Design review of the part built by this model. Coordinates are the model's own, in mm. Face numbers are marked on the shaded views. A direction names the side the tool comes from. Give positions to 0.01 mm unless a question says otherwise; leave off trailing zeros. Loops run counter-clockwise (first coordinate to the right, second up) from the corner with the lowest first, then second, coordinate; pieces in that order, holes last.
Autodesk Inventor part; units mm, degrees
ref_plane "YZ Plane" through (0, 0, 0) normal (1, 0, 0) x (0, 1, 0)
ref_plane "XZ Plane" through (0, 0, 0) normal (0, 1, 0) x (-1, 0, 0)
ref_plane "XY Plane" through (0, 0, 0) normal (0, 0, 1) x (1, 0, 0)
sketch "Sketch1" plane through (0, 0, 0) normal (0, 0, 1) x (1, 0, 0)
  arc A0 (1.7145, 0) -> (-1.7145, 0) centre (0, 0) ccw
  arc A1 (38.0096, -20.955) -> (34.5806, -20.955) centre (36.2951, -20.955) ccw
  line L0 (0, 0) -> (36.5724, 0) construction
  line L1 (-1.7145, 0) -> (-1.7145, -3.0427)
  line L2 (1.7145, 0) -> (1.7145, -3.0427)
  line L3 (34.5806, -20.955) -> (34.5806, -23.9977)
  line L4 (38.0096, -20.955) -> (38.0096, -23.9977)
  line L5 (0, 0) -> (0, -41.91) construction
  arc A2 (29.1702, -5.2325) -> (5.0807, 4.6768) centre (0, -41.91) ccw
  arc A3 (5.0807, 4.6768) -> (-2.0016, 2.862) centre (3.9541, -5.6536) ccw
  arc A4 (39.5833, -19.7781) -> (29.1702, -5.2325) centre (8.8547, -30.7765) ccw
  arc A5 (4.8053, 2.1517) -> (2.7829, 2.1102) centre (3.9541, -5.6536) ccw
  arc A6 (27.5892, -7.2205) -> (4.8053, 2.1517) centre (0, -41.91) ccw
  arc A7 (35.8607, -17.4896) -> (27.5892, -7.2205) centre (8.8547, -30.7765) ccw
  arc A8 (35.8607, -17.4896) -> (34.5806, -23.9977) centre (36.2951, -20.955) ccw
  arc A9 (38.0096, -23.9977) -> (39.5833, -19.7781) centre (36.2951, -20.955) ccw
  arc A10 (-2.0016, 2.862) -> (-1.7145, -3.0427) centre (0, 0) ccw
  arc A11 (1.7145, -3.0427) -> (2.7829, 2.1102) centre (0, 0) ccw
  line L6 (0, 0) -> (36.2951, -20.955) construction
  line L7 (12.8786, -1.5696) -> (6.5286, -12.5681)
  line L8 (6.5286, -12.5681) -> (22.1465, -21.5851)
  line L9 (22.1465, -21.5851) -> (28.4965, -10.5866)
  line L10 (28.4965, -10.5866) -> (12.8786, -1.5696)
  line L11 (28.4965, -10.5866) -> (36.2951, -20.955) construction
  line L12 (12.8786, -1.5696) -> (0, 0) construction
  line L13 (12.8786, -1.5696) -> (13.8891, 0.1806)
  line L14 (28.4965, -10.5866) -> (29.4898, -8.8662)
  line L15 (15.0783, -2.8396) -> (8.7283, -13.8381)
  line L16 (26.2968, -9.3166) -> (19.9468, -20.3151)
  dimension "d0" = 3.429
  dimension "d1" = 30
  dimension "d3" = 41.91
  dimension "d4" = 93.726
  dimension "d6" = 2.54
  dimension "d7" = 5.08
  dimension "d8" = 18.034
  dimension "d9" = 41.91
  dimension "d10" = 6.985
  dimension "d11" = 12.7
  dimension "d12" = 2.54
  dimension "d13" = 2.54
  dimension "d14" = 3.429
  dimension "d15" = 3.4925
extrude "Extrusion1" add sketch "Sketch1" along normal blind 4.445
fillet "Fillet1" radius 2.54 4 edges at (2.7829, 2.1102, 2.2225) (35.8607, -17.4896, 2.2225) (29.4898, -8.8662, 2.2225) (13.8891, 0.1806, 2.2225)
fillet "Fillet2" radius 0.381 4 edges at (-1.7145, -3.0427, 2.2225) (1.7145, -3.0427, 2.2225) (34.5806, -23.9977, 2.2225) (38.0096, -23.9977, 2.2225)
extrude "Extrusion2" add sketch "Sketch1" along normal blind 7.239 contours L10 L15 L8 L7 | L9 L8 L16 L10
properties part number "USBBreakoutHolder"
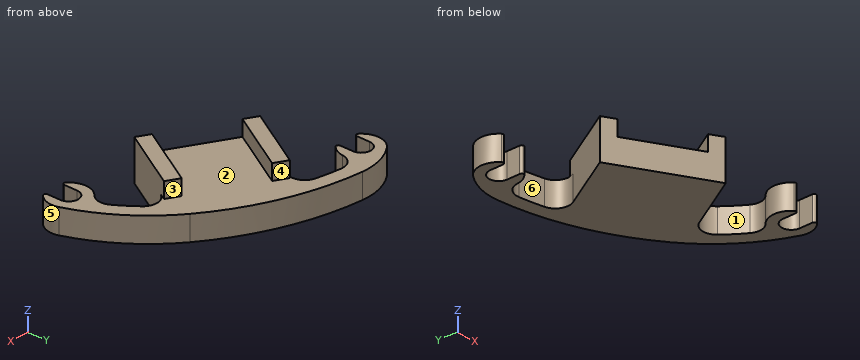
Q1. Take a section at B-B (x = 17). Give the boundary of the cut face in (y, z) (3 decimals), plus the area to 3 significant figures.
Results:
outline: (-18.614, 0) - (1.761, 0) - (1.761, 4.445) - (-18.614, 4.445) - close
area: 90.6 mm2
Q2. Tool access review of the marked faces 4, 5 and 6: name each direction out of +Z, -Z, +X, -X, +Y, -Y from which nothing blocks a thin tool from reaching the whole face with its end or side.
Results:
face 4: +Z, +X, +Y
face 5: +Z, -Z, +X
face 6: +Z, -Z
Q3. Wall thickness on line 1 (X direction, y = -19.5, z = 2.5) (3 decimals); line 2 (X direction, y = -22, z = 1.75); line 3 (Z direction, x = 28, y = -8) (3 decimals): over which ranges is each line inside the solid? List them lowest first.
Results:
line 1: x = 18.535 to 23.35, 33.12 to 35.388, 37.202 to 39.482
line 2: x = 32.96 to 34.58, 38.01 to 39.63
line 3: z = 0 to 4.445
Q4. Take a section at A-A (x = 0). Give the boundary of the cut face in (y, z) (1 decimal), plus the area to 3 significant figures.
Results:
outline: (1.7, 0) - (4, 0) - (4, 4.4) - (1.7, 4.4) - close
area: 9.97 mm2
Q5. Insertion check: pin 1 (1.2 mm diameter, centred on y = -1.5, z = 2, fed in from +X); pin 2 (3 mm diameter, centred on x = 8, z = 1.5, fed in from -Y); pin 3 (4 mm diameter, centred on x = 7.5, z = 6.5, fed in from +Y); pin 4 (3 mm diameter, centred on x = 22, y = -8, fed in from -Z). Each pin has a flat end and moves straight along its axis. Give the tip position at first contact, or say it passes through.
Results:
pin 1: stops at x = 24.72
pin 2: stops at y = -14.28
pin 3: stops at y = -7.42
pin 4: stops at z = 0
Q6. Draft analysis for pull direction Y (two halves, no side actions). For the marked faces 1, 2 and 3, state which applies: pulls with the +Y half, pulls with the -Y half, needs draft (parallel to the pull), parting line crosses it, or undercut.
Results:
face 1: undercut
face 2: needs draft
face 3: pulls with the +Y half
